Could you check a few things on this drawing? It's one solid part, dimensions in mm from its lowest x, y, z. Coordinates: 2 decimals unless noted, no trailing zeros. Write each loop counter-clockwise with the first axis right and the second up, starting at its lowest first coordinate (ties: lowest second). Pieces come first, ordered by that corner, then holes. Notation, with made-up numbers: (73, 50.25) - (108, 50.25) arc R30 ccw to (108, 75.25) - close; hole circle Ø1 at (75, 36). An arc over 180 degrees is marked (long way). Answer as a JSON object with one key per item and string values. Group by question number.
1) Will these pins go through, and if not, where does the flat tip stop? pin 1 Ø12 at (y, z) = (45, 8) entering from -X; pin 2 Ø1 at (x, z) = (20.5, 20.5) entering from +Y; pin 3 Ø1.5 at (x, z) = (25.5, 15) entering from +Y.
2) Please list where these lines run through material, in increasing order: line 1 along Y through (x, z) = (25, 26.7); line 2 along Y through (x, z) = (25, 19); line 3 along Z through (x, y) = (43.5, 22.5).
3) We'd pull the mould along Y, two halves only. Please class the marked faces 1, 2, 3 and 4: released by +Y, released by -Y, zero draft, split by the parting line, or undercut.
4) If we section it at C-C (z = 25.75): Write out the boundary of the cut face in (x, y).
5) If we section it at A-A (y = 25): Write out the boundary of the cut face in (x, z).
6) If we section it at D-D (x = 7): Write out the boundary of the cut face in (y, z), plus the area to 3 significant figures.
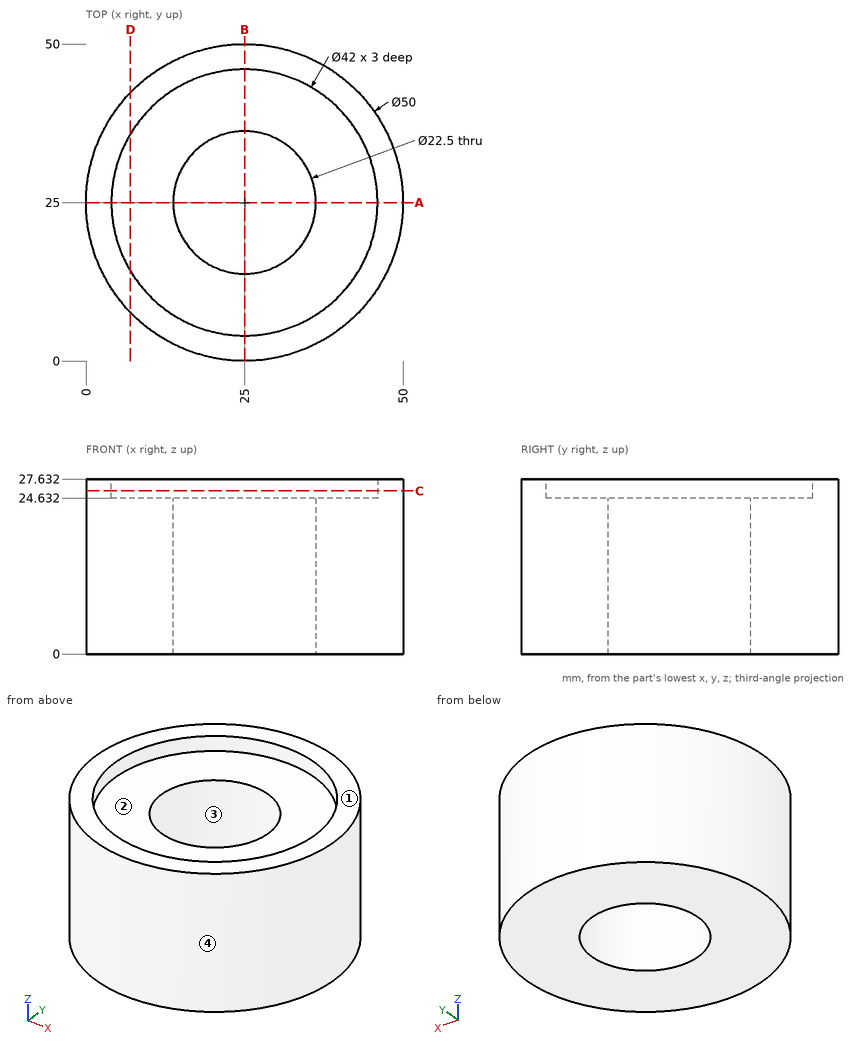
Here are the results:
{
 "1": {"pin 1": "stops at x = 4.29", "pin 2": "stops at y = 49.68", "pin 3": "stops at y = 50"},
 "2": {"line 1": "y = 0 to 4, 46 to 50", "line 2": "y = 0 to 13.75, 36.25 to 50", "line 3": "z = 0 to 24.63"},
 "3": {"face 1": "zero draft", "face 2": "undercut", "face 3": "undercut", "face 4": "split by the parting line"},
 "4": {"outline": "circle Ø50 at (25, 25); hole circle Ø42 at (25, 25)"},
 "5": {"outline": "(0, 0) - (13.75, 0) - (13.75, 24.63) - (4, 24.63) - (4, 27.63) - (0, 27.63) - close; (36.25, 0) - (50, 0) - (50, 27.63) - (46, 27.63) - (46, 24.63) - (36.25, 24.63) - close"},
 "6": {"outline": "(7.65, 0) - (42.35, 0) - (42.35, 27.63) - (35.82, 27.63) - (35.82, 24.63) - (14.18, 24.63) - (14.18, 27.63) - (7.65, 27.63) - close", "area": "894 mm²"}
}
